```python
from build123d import *

# Parameters (mm, degrees)
SKETCH1_W           = 7.62
SKETCH1_H           = 20.447
BOSS_EXTRUDE1_DEPTH = 1.016
SKETCH2_W           = 7.62
SKETCH2_H           = 3.175
BOSS_EXTRUDE2_DEPTH = 6.35
SKETCH3_R           = 1.905
CUT_EXTRUDE1_DEPTH  = 22.746687311
SKETCH5_W           = 7.62
SKETCH5_H           = 7.62
SKETCH5_W_2         = 6.223
SKETCH5_H_2         = 6.223
BOSS_EXTRUDE3_DEPTH = 3.302
CUT_EXTRUDE3_DEPTH  = 14.16411821


with BuildPart() as part:
    # Sketch1 → Boss-Extrude1 (new body)
    with BuildSketch(Plane.XY):
        Rectangle(SKETCH1_W, SKETCH1_H)
    extrude(amount=BOSS_EXTRUDE1_DEPTH)

    # Sketch2 → Boss-Extrude2 (add)
    with BuildSketch(Plane(origin=(0, 0, 0), x_dir=(-1, 0, 0), z_dir=(0, 0, -1))):
        with Locations((0, 8.636)):
            Rectangle(SKETCH2_W, SKETCH2_H)
        with Locations((0, -1.143)):
            Rectangle(SKETCH2_W, SKETCH2_H)
    extrude(amount=BOSS_EXTRUDE2_DEPTH)

    # Sketch3 → Cut-Extrude1 (cut, through all)
    with BuildSketch(Plane(origin=(0, 10.2235, 0), x_dir=(1, 0, 0), z_dir=(0, 1, 0))):
        with Locations(Location((0, 3.302, 0), (0, 0, 180))):
            Circle(SKETCH3_R)
    extrude(amount=-CUT_EXTRUDE1_DEPTH, mode=Mode.SUBTRACT)

    # Sketch5 → Boss-Extrude3 (add)
    with BuildSketch(Plane.XY.offset(1.016)):
        with Locations((0, -6.4135)):
            Rectangle(SKETCH5_W, SKETCH5_H)
        with Locations((0, -6.39034895)):
            Rectangle(SKETCH5_W_2, SKETCH5_H_2, mode=Mode.SUBTRACT)
    extrude(amount=BOSS_EXTRUDE3_DEPTH)

    # Sketch7 → Cut-Extrude3 (cut, through all)
    with BuildSketch(Plane.XY.offset(1.016)):
        Polygon((-3.1115, -7.91434895), (-1.524, -7.91434895), (1.524, -7.91434895), (3.1115, -7.91434895), (3.1115, -4.86634895), (1.524, -4.86634895), (-1.524, -4.86634895), (-3.1115, -4.86634895), align=None)
    extrude(amount=-CUT_EXTRUDE3_DEPTH, mode=Mode.SUBTRACT)


solid = part.part
```
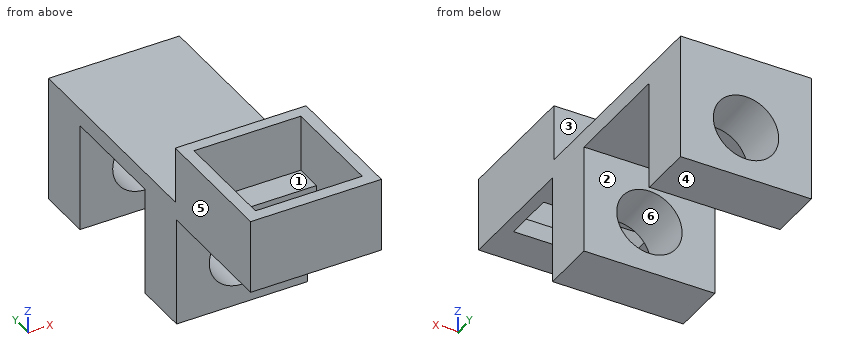
Geometry: final body of the model. Coordinates: model frame, mm. Face numbers are marked on the shaded views. A direction names the side the tool comes from. Give positions to 0.01 mm unless a question says otherwise; leave off trailing zeros. Write each loop counter-clockwise with the first axis right and the second up, starting at its lowest first coordinate (ties: lowest second). Pieces come first, ordered by that corner, then holes.
1. Reachability of the marked faces 1, 2 and 3 from +Z, -Z, +X, -X, +Y, -Y: full face, straight path, thin tool, end or side. Return the list, or none.
2. Section query A-A, the plane y = -6.75. Return loops of the section in (x, z).
3. Section query B-B, the plane z = -0.5. Return loops of the section in (x, y).
4. Draft query along X for the marked faces 4, 5 and 6. Return one class per face: released by +X, released by -X, zero draft, split by the parting line, or undercut.
5. Section query D-D, the plane z = 2. Return loops of the section in (x, y).
6. Pin query (flat end, axial travel): P1, Ø0.5, axis at x = -1, y = -9, coming from the +Z side; P2, Ø3.5, axis at x = 0, z = 3.5, coming from the +Y side; P3, Ø2, axis at x = -1.5, y = -7, coming from the -Z side. Return the tip coordinate at first contact, or that it passes through.
7. Line query: probe 1 along Y at (x, z) = (0.25, -0.25); probe 2 along X at (y, z) = (-6, 4.25); probe 3 along Y at (x, z) = (2, 1.75). Output: solid intervals per line, ascending.
8. Section query C-C, the plane x = 0. Return loops of the section in (y, z).
Computed:
1. face 1: +Z
1. face 2: -Z, +X, -X
1. face 3: +Z, +X, -X, +Y
2. outline: (-3.81, 0) - (-3.11, 0) - (-3.11, 4.32) - (-3.81, 4.32) - close; (3.11, 0) - (3.81, 0) - (3.81, 4.32) - (3.11, 4.32) - close
3. outline: (-3.81, -2.73) - (3.81, -2.73) - (3.81, 0.44) - (-3.81, 0.44) - close; (-3.81, 7.05) - (3.81, 7.05) - (3.81, 10.22) - (-3.81, 10.22) - close
4. face 4: zero draft
4. face 5: released by -X
4. face 6: undercut
5. outline: (-3.81, -10.22) - (3.81, -10.22) - (3.81, -2.6) - (-3.81, -2.6) - close; hole (-3.11, -9.5) - (3.11, -9.5) - (3.11, -3.28) - (-3.11, -3.28) - close
6. P1: stops at z = 1.02
6. P2: stops at y = -2.6
6. P3: stops at z = 0
7. probe 1: y = -2.73 to 0.44, 7.05 to 10.22
7. probe 2: x = -3.81 to -3.11, 3.11 to 3.81
7. probe 3: y = -10.22 to -9.5, -3.28 to -2.6
8. outline: (-10.22, 0) - (-7.91, 0) - (-7.91, 1.02) - (-9.5, 1.02) - (-9.5, 4.32) - (-10.22, 4.32) - close; (-4.87, 0) - (-2.73, 0) - (-2.73, -1.4) - (0.44, -1.4) - (0.44, 0) - (7.05, 0) - (7.05, -1.4) - (10.22, -1.4) - (10.22, 1.02) - (-2.6, 1.02) - (-2.6, 4.32) - (-3.28, 4.32) - (-3.28, 1.02) - (-4.87, 1.02) - close; (-2.73, -6.35) - (0.44, -6.35) - (0.44, -5.21) - (-2.73, -5.21) - close; (7.05, -6.35) - (10.22, -6.35) - (10.22, -5.21) - (7.05, -5.21) - close
